```python
from build123d import *

# Parameters (mm, degrees)
F0_W     = 76.2
F0_H     = 76.2
F1_DEPTH = 3.175
F4_DEPTH = 76.2
F5_DEPTH = 76.2


with BuildPart() as f1:
    # F0 (on Top) → F1 (new body)
    with BuildSketch(Plane.XY):
        Rectangle(F0_W, F0_H)
    extrude(amount=F1_DEPTH)

    # F3 (on face) → F4 (cut)
    with BuildSketch(Plane(origin=(0, 38.1, 0), x_dir=(-1, 0, 0), z_dir=(0, 1, 0))):
        Polygon((-38.1, 3.175), (-38.1, 0), (-34.925, 3.175), align=None)
        Polygon((34.925, 3.175), (38.1, 0), (38.1, 3.175), align=None)
    extrude(amount=-F4_DEPTH, mode=Mode.SUBTRACT)

    # F2 (on face) → F5 (cut)
    with BuildSketch(Plane.YZ.offset(38.1)):
        Polygon((34.925, 3.175), (38.1, 0), (38.1, 3.175), align=None)
        Polygon((-38.1, 3.175), (-38.1, 0), (-34.925, 3.175), align=None)
    extrude(amount=-F5_DEPTH, mode=Mode.SUBTRACT)


solid = f1.part
```
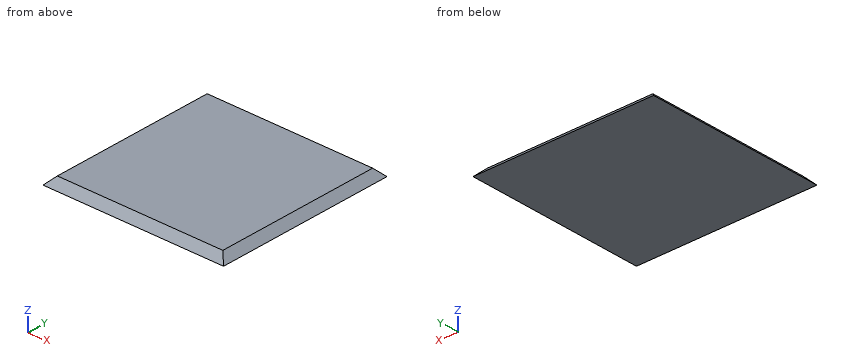
The listing builds one solid part. Answer for the finished solid, in the listing's coordinates (mm). Round coordinates to 2 decimals unless told otherwise and drop trailing zeros. Order: outer loops, then holes, each group sorted by start corner. A loop starts at its lowest first (then second) coordinate and runs counter-clockwise, first axis right, second up. Notation, with made-up numbers: (-8.75, -19.5) - (26.25, -19.5) arc R10 cw to (26.25, -4.5) - close; hole circle Ø2 at (-31.5, 59). An arc over 180 degrees is marked (long way). Put each result on its own line as item: value. Start each with the question number.
(1) Find section A-A (z = 2.5). Give the vertices of the cut face in (x, y).
(2) Find section B-B (x = 31.5). Give the vertices of the cut face in (y, z) (3 decimals), plus the area to 3 significant figures.
(3) Straight lines are drawn through the part: probe 1 along X at (y, z) = (-4, 0.6); probe 2 along X at (y, z) = (-9, 0.3); probe 3 along Y at (x, z) = (-9, 3.05). For each, find the intervals that lie inside material, in ascending order. Write a range as from..to.
Reply:
1. outline: (-35.6, -35.6) - (35.6, -35.6) - (35.6, 35.6) - (-35.6, 35.6) - close
2. outline: (-38.1, 0) - (38.1, 0) - (34.925, 3.175) - (-34.925, 3.175) - close
2. area: 232 mm^2
3. probe 1: -37.5..37.5
3. probe 2: -37.8..37.8
3. probe 3: -35.05..35.05
